Verification items for the finished model (mm, model axes). Face numbers are marked on the shaded views. A direction names the side the tool comes from. Give positions to 0.01 mm unless a question says otherwise; leave off trailing zeros. Write each loop counter-clockwise with the first axis right and the second up, starting at its lowest first coordinate (ties: lowest second). Pieces come first, ordered by that corner, then holes. Notation, with made-up numbers: (-16.5, -12) -> (21.5, -12) arc R35 ccw to (21.5, 24) -> close; hole circle Ø10 at (68.5, 23). An arc over 180 degrees is marked (long way). Answer as CSV lines item,"result".
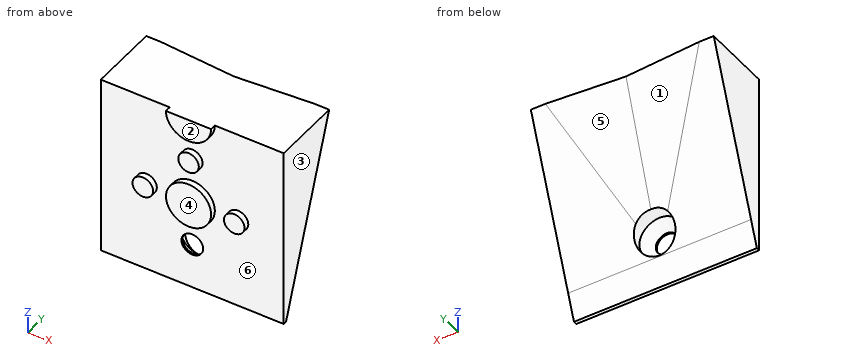
```python
from build123d import *

# Parameters (mm, degrees)
BOSS_EXTRUDE1_DEPTH = 16
BOSS_EXTRUDE2_REACH = 12.077
SKETCH6_W           = 32
SKETCH6_H           = 7.878
SKETCH6_R           = 3.5433
SKETCH7_R           = 1.7992
SKETCH7_R_2         = 3.9492
BOSS_EXTRUDE3_DEPTH = 1.016
CUT_EXTRUDE1_DEPTH  = 34.720378775


with BuildPart() as part:
    # Sketch1 → Boss-Extrude1 (new body, symmetric)
    with BuildSketch(Plane(origin=(0, 0, 0), x_dir=(0, 0, -1), z_dir=(1, 0, 0))):
        Polygon((19.808, 5.059429759), (19.808, 2.192072254), (27.686, 2.192072254), (32, 0.621904663), (32, 0), (0, 0), (0, 12.26895216), align=None)
    extrude(amount=BOSS_EXTRUDE1_DEPTH, both=True)

    # Sketch5 → CSK for _6 Flat Head Machine Screw1 (revolve, cut)
    with BuildSketch(Plane(origin=(0, 2.192072254, -24), x_dir=(0, 0, 1), z_dir=(1, 0, 0))):
        Polygon((0, 0), (0, 2.192072254), (1.89865, 2.192072254), (1.89865, 1.891953401), (3.5433, 0), align=None)
    revolve(axis=Axis((0, 8.542072254, -24), (0, -1, 0)), mode=Mode.SUBTRACT)

    # Boss-Extrude2: up to this face of the body (flat: up to its plane)
    boss_extrude2_end = Plane(part.part.faces().sort_by_distance((0, 8.664190959, -9.904))[0])
    # Sketch6 → Boss-Extrude2 (add, up to the picked face)
    with BuildSketch(Plane(origin=(0, 2.192072254, 0), x_dir=(1, 0, 0), z_dir=(0, 1, 0)), mode=Mode.PRIVATE) as boss_extrude2_sk1:
        with Locations((0, 23.747)):
            Rectangle(SKETCH6_W, SKETCH6_H)
        with Locations((0, 24)):
            Circle(SKETCH6_R, mode=Mode.SUBTRACT)
    boss_extrude2_tool1 = split(extrude(boss_extrude2_sk1.sketch, amount=BOSS_EXTRUDE2_REACH, mode=Mode.PRIVATE), bisect_by=boss_extrude2_end, keep=Keep.BOTH, mode=Mode.PRIVATE)
    add(boss_extrude2_tool1.solids().sort_by_distance((-15.670445, 2.192072, -23.747))[0])

    # Sketch7 → Boss-Extrude3 (add)
    with BuildSketch(Plane.XZ):
        with Locations((8, -16)):
            Circle(SKETCH7_R)
        with Locations((0, -16)):
            Circle(SKETCH7_R_2)
        with Locations((-8, -16)):
            Circle(SKETCH7_R)
        with Locations((0, -8)):
            Circle(SKETCH7_R)
        with BuildLine():
            Line((3.9492, 0), (-3.9492, 0))
            ThreePointArc((-3.9492, 0), (0, -3.9492), (3.9492, 0))
        make_face()
    extrude(amount=BOSS_EXTRUDE3_DEPTH)

    # Sketch9 → Cut-Extrude1 (cut, through all, along a direction that is not the sketch's normal)
    with BuildSketch(Plane.XY):
        Polygon((-13.46, 12.26895216), (0, 11.25295216), (13.46, 12.26895216), align=None)
    extrude(amount=-CUT_EXTRUDE1_DEPTH, dir=(0, 0.310876055, 0.950450461), mode=Mode.SUBTRACT)


solid = part.part
```
1) Section check D-D (z = -13). Record the boundary of the cut face in (x, y).
Reported:
outline,"(-16, 0) -> (-2.57, 0) -> (-2.57, -1.02) -> (2.57, -1.02) -> (2.57, 0) -> (16, 0) -> (16, 7.54) -> (7.11, 7.54) -> (0, 7) -> (-7.11, 7.54) -> (-16, 7.54) -> close"
2) Depth check by flat-ended pin: pin 1 (8 mm diameter, centred on x = -12.5, z = -22.5, fed in from +Y); pin 2 (6 mm diameter, centred on x = 0, z = -24, fed in from -Y). Enter the tip coordinate at first touch or a pass-through.
Reported:
pin 1,"y = 5.54"
pin 2,"y = 0"
3) Section check B-B (x = 8). Record the boundary of the cut face in (y, z), and give its area (3 significant figures).
Reported:
outline,"(-1.02, -17.8) -> (0, -17.8) -> (0, -32) -> (0.62, -32) -> (8.2, -11.17) -> (11.86, 0) -> (0, 0) -> (0, -14.2) -> (-1.02, -14.2) -> close"
area,"208 mm²"
4) Section check C-C (y = 5.5). Record the boundary of the cut face in (x, z), and give its area (3 significant figures).
Reported:
outline,"(-16, -18.6) -> (-4.37, -18.6) -> (0, -17.59) -> (4.37, -18.6) -> (16, -18.6) -> (16, 0) -> (-16, 0) -> close"
area,"591 mm²"
5) Tool access check on the marked faces 4, 5 and 6. Record the directions out of +Z, -Z, +X, -X, +Y, -Y that give a thin tool (end or side, any length) a straight path to the whole face; none if there is none.
Reported:
face 4,"+Z, -Z, +X, -X, -Y"
face 5,"-Z, +Y"
face 6,"-Y"
6) Draft check along X on the marked faces 1, 2 and 3. Enter one of: +X half, -X half, draft (parallel to the pull), parting line (faces both ways), or undercut.
Reported:
face 1,"undercut"
face 2,"draft"
face 3,"+X half"
7) Section check A-A (z = -24). Record the boundary of the cut face in (x, y).
Reported:
outline,"(-16, 0) -> (-1.9, 0) -> (-1.9, 0.3) -> (-3.54, 2.19) -> (-3.54, 3.53) -> (-16, 3.53) -> close; (1.9, 0) -> (16, 0) -> (16, 3.53) -> (3.54, 3.53) -> (3.54, 2.19) -> (1.9, 0.3) -> close"
8) Scan lines: line 1 along X through (y, z) = (0.15, -24); line 2 along Z through (x, y) = (0, 0.15); line 3 along Z through (x, y) = (0, 3.5). Record each from-to range of solid material in increasing order.
Reported:
line 1,"-16 to -1.9, 1.9 to 16"
line 2,"-32 to -25.9, -22.1 to 0"
line 3,"-20.46 to 0"
